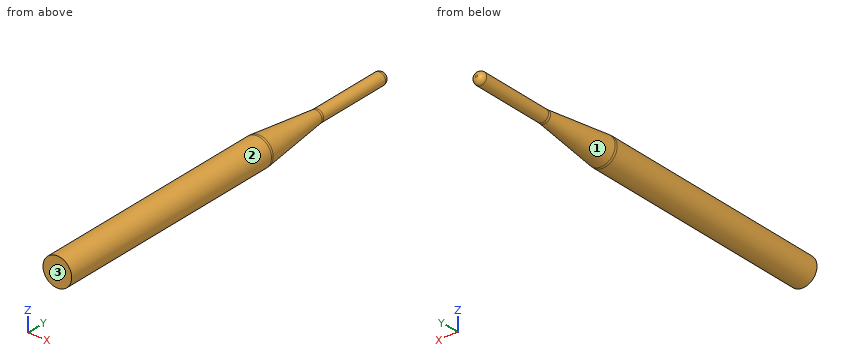
from build123d import *


with BuildPart() as part:
    # Sketch2 → Antenna (revolve)
    with BuildSketch(Plane.XY, mode=Mode.PRIVATE) as antenna_sk:
        with BuildLine():
            Line((3, 192.5), (3, 155.569574769))
            ThreePointArc((3, 155.569574769), (3.01618141, 155.000921652), (3.064673273, 154.434108857))
            Line((3.064673273, 154.434108857), (6.935326727, 120.565891143))
            ThreePointArc((6.935326727, 120.565891143), (6.98381859, 119.999078348), (7, 119.430425231))
            Line((7, 119.430425231), (7, 0))
            Line((7, 0), (0, 0))
            Line((0, 0), (0, 195))
            Line((0, 195), (0.5, 195))
            ThreePointArc((0.5, 195), (2.267766953, 194.267766953), (3, 192.5))
        make_face()
    revolve(antenna_sk.sketch.rotate(Axis((0, 0, 0), (0, 1, 0)), 90), axis=Axis((0, 0, 0), (0, 1, 0)))


solid = part.part
Read the model definition and answer for the solid it produces. Units are mm, in the model's axes. Face numbers are marked on the shaded views. Give positions to 0.01 mm unless a question says otherwise; leave off trailing zeros. Write each loop counter-clockwise with the first axis right and the second up, starting at its lowest first coordinate (ties: lowest second). Pieces come first, ordered by that corner, then holes. Notation, with made-up numbers: (0.25, 33.25) - (55.25, 33.25) arc R34 ccw to (55.25, 64.25) - close; hole circle Ø5 at (-24, 32). An arc over 180 degrees is marked (long way). Return JSON: item names as keys, results as strings.
Q1. Consider line 1 along Z through (x, y) = (-0.75, 11); line 2 along X through (y, z) = (96.5, 1). Determine where each line is inside the solid, lowest interval first. Write a range as [from, to].
Reply:
{"line 1": "[-6.96, 6.96]", "line 2": "[-6.93, 6.93]"}
Q2. Given P1, Ø5, axis at y = 42.5, z = -4, coming from the -X side, flat-ended and moving along its own axis, determine where the tip first touches the part or whether it passes through.
Reply:
{"P1": "x = -6.84"}
Q3. A cutting plane is placed at A-A, the plane y = 174.5. Determine the outline of the cut face in (x, z), and give its area (3 significant figures).
Reply:
{"outline": "circle Ø6 at (0, 0)", "area": "28.3 mm²"}
Q4. A cutting plane is placed at B-B, the plane y = 82. Determine the outline of the cut face in (x, z), and give its area (3 significant figures).
Reply:
{"outline": "circle Ø14 at (0, 0)", "area": "154 mm²"}
Q5. For a pull along Y with two mould halves and no side action, classify the marked faces 1, 2 and 3 as released by +Y, released by -Y, zero draft, split by the parting line, or undercut.
Reply:
{"face 1": "released by +Y", "face 2": "zero draft", "face 3": "released by -Y"}
